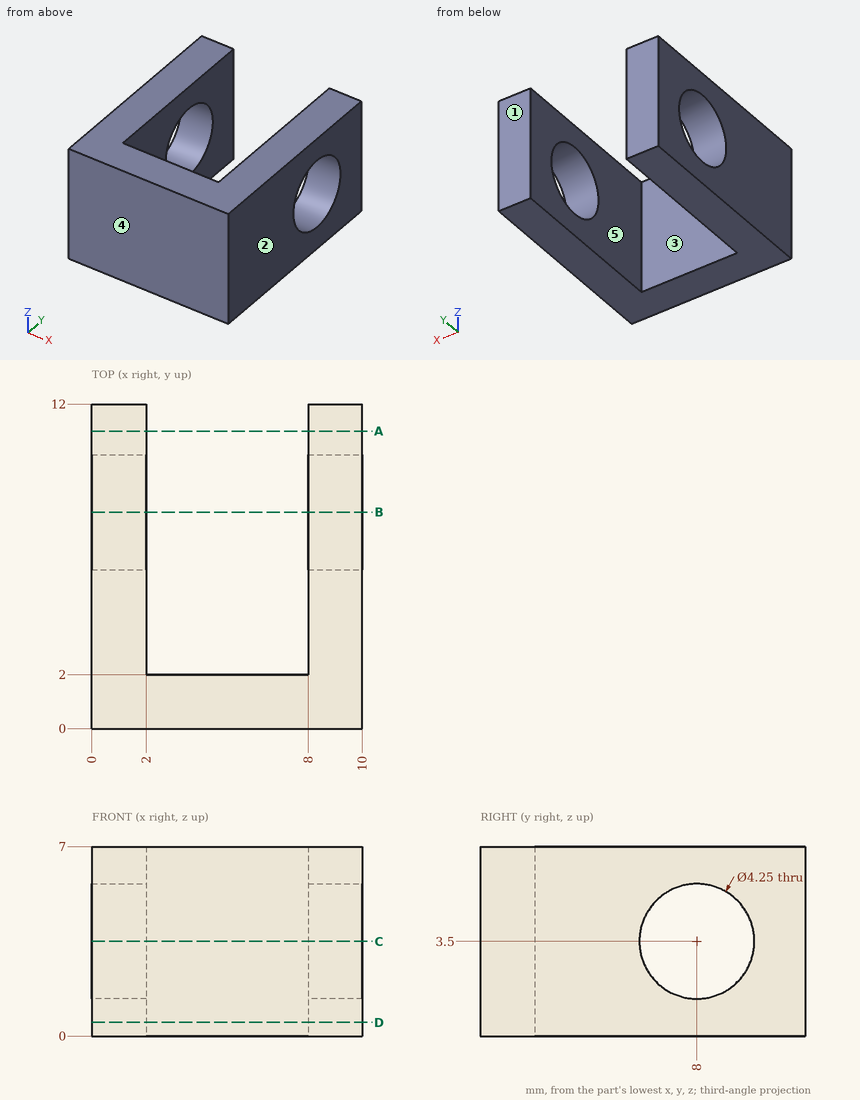
Can you work these out from the drawing? Everything is in mm from the part's minimum corner. A direction names the side the tool comes from. Give positions to 0.01 mm unless a question says otherwise; leave off trailing zeros. Loops run counter-clockwise (first coordinate to the right, second up) from the corner with the lowest first, then second, coordinate; pieces in that order, holes last. Notation, with made-up numbers: (20.25, 82.5) -> (59.25, 82.5) arc R20 cw to (59.25, 99.5) -> close; hole circle Ø4 at (81.25, 66.5). An arc over 180 degrees is marked (long way). Return JSON: item names as keys, results as strings.
Q1. I want a section at A-A, the plane y = 11. List the corners of the cut face in (x, z) for me.
Checks:
{"outline": "(0, 0) -> (2, 0) -> (2, 7) -> (0, 7) -> close; (8, 0) -> (10, 0) -> (10, 7) -> (8, 7) -> close"}
Q2. I need wall thicknesses on probe 1 along X at (y, z) = (7.75, 1); probe 2 along Y at (x, z) = (0.75, 3.5) (3 decimals); probe 3 along Y at (x, z) = (2.25, 2.5). Which ranges of each line are inside material? Lowest first, please.
Checks:
{"probe 1": "x = 0 to 2, 8 to 10", "probe 2": "y = 0 to 5.875, 10.125 to 12", "probe 3": "y = 0 to 2"}
Q3. For pin 1 Ø2 at (x, z) = (6, 4.5) entering from +Y, with a flat end and sliding along its axis, tell me the tip position at first contact or that it passes through.
Checks:
{"pin 1": "stops at y = 2"}
Q4. I want a section at B-B, the plane y = 8. List the corners of the cut face in (x, z) for me (3 decimals), then the cut area to 3 significant figures.
Checks:
{"outline": "(0, 0) -> (2, 0) -> (2, 1.375) -> (0, 1.375) -> close; (0, 5.625) -> (2, 5.625) -> (2, 7) -> (0, 7) -> close; (8, 0) -> (10, 0) -> (10, 1.375) -> (8, 1.375) -> close; (8, 5.625) -> (10, 5.625) -> (10, 7) -> (8, 7) -> close", "area": "11.0 mm2"}
Q5. I want a section at D-D, the plane z = 0.5. List the corners of the cut face in (x, y) for me, then the cut area to 3 significant figures.
Checks:
{"outline": "(0, 0) -> (10, 0) -> (10, 12) -> (8, 12) -> (8, 2) -> (2, 2) -> (2, 12) -> (0, 12) -> close", "area": "60.0 mm2"}
Q6. We'd pull the mould along X, two halves only. Please class the marked faces 1, 2 and 3: released by +X, released by -X, zero draft, split by the parting line, or undercut.
Checks:
{"face 1": "zero draft", "face 2": "released by +X", "face 3": "undercut"}
Q7. I want a section at C-C, the plane z = 3.5. List the corners of the cut face in (x, y) for me (3 decimals), then the cut area to 3 significant figures.
Checks:
{"outline": "(0, 0) -> (10, 0) -> (10, 5.875) -> (8, 5.875) -> (8, 2) -> (2, 2) -> (2, 5.875) -> (0, 5.875) -> close; (0, 10.125) -> (2, 10.125) -> (2, 12) -> (0, 12) -> close; (8, 10.125) -> (10, 10.125) -> (10, 12) -> (8, 12) -> close", "area": "43.0 mm2"}
Q8. On a 3-axis mill with a long thin cutter (end or side, diameter ignored), from which of +Z, -Z, +X, -X, +Y, -Y can I reach the whole of each face in a straight line? I mean the marked faces 4 and 5. Say none if no direction works.
Checks:
{"face 4": "+Z, -Z, +X, -X, -Y", "face 5": "+Z, -Z, +Y"}
